Check sheet for the modelled part. Datum: model origin and axes. Units: mm. A direction names the side the tool comes from. Give positions to 0.01 mm unless a question says otherwise; leave off trailing zeros. Order: outer loops, then holes, each group sorted by start corner. A loop starts at its lowest first (then second) coordinate and runs counter-clockwise, first axis right, second up.
```python
from build123d import *

# Parameters (mm, degrees)
SKETCH1_R           = 69.85
BOSS_EXTRUDE1_DEPTH = 177.8
SKETCH2_R           = 25.4
CUT_EXTRUDE1_DEPTH  = 204.398340701
SKETCH3_R           = 63.5
CUT_EXTRUDE2_DEPTH  = 165.1


with BuildPart() as part:
    # Sketch1 → Boss-Extrude1 (new body)
    with BuildSketch(Plane.XY):
        Circle(SKETCH1_R)
    extrude(amount=BOSS_EXTRUDE1_DEPTH)

    # Sketch2 → Cut-Extrude1 (cut, through all)
    with BuildSketch(Plane.XY.offset(177.8)):
        Circle(SKETCH2_R)
    extrude(amount=-CUT_EXTRUDE1_DEPTH, mode=Mode.SUBTRACT)

    # Sketch3 → Cut-Extrude2 (cut)
    with BuildSketch(Plane.XY.offset(177.8)):
        Circle(SKETCH3_R)
    extrude(amount=-CUT_EXTRUDE2_DEPTH, mode=Mode.SUBTRACT)


solid = part.part
```
(1) Cross-section at A-A on x = 0. Enter the section's corners in (y, z).
Response values:
outline: (-69.85, 0) - (-25.4, 0) - (-25.4, 12.7) - (-63.5, 12.7) - (-63.5, 177.8) - (-69.85, 177.8) - close; (25.4, 0) - (69.85, 0) - (69.85, 177.8) - (63.5, 177.8) - (63.5, 12.7) - (25.4, 12.7) - close
(2) Release check for a two-part mould opening along X. For faces 1 (the face through (30, 1, 0)), 2 (the face through (-55.431, -42.503, 87.655)), 3 (the face through (27, 1, 12.7)) record: released by +X, released by -X, zero draft, split by the parting line, or undercut.
Response values:
face 1: zero draft
face 2: split by the parting line
face 3: undercut
(3) Set-up check for faces 4 (the face through (15, -62, 177.8)), 5 (the face through (-13.77, -61.99, 96.41)): record each of +Z, -Z, +X, -X, +Y, -Y from which the full face is reachable in a straight line by a thin tool's end or side.
Response values:
face 4: +Z, +X, -X, +Y, -Y
face 5: +Z
(4) Cross-section at D-D on y = -39.5. Enter the section's corners in (x, z).
Response values:
outline: (-57.61, 0) - (57.61, 0) - (57.61, 177.8) - (49.72, 177.8) - (49.72, 12.7) - (-49.72, 12.7) - (-49.72, 177.8) - (-57.61, 177.8) - close
(5) Gauge pin test, flat ends, axial feed: pin 1 Ø1 at (x, z) = (-27.5, 145) entering from +Y; pin 2 Ø6 at (x, z) = (47, 19) entering from -Y; pin 3 Ø4 at (x, z) = (-25, 147) entering from -Y. Record the tip position at first contact, or that the pin passes through.
Response values:
pin 1: stops at y = 64.42
pin 2: stops at y = -54.25
pin 3: stops at y = -65.95
(6) Material ranges on L1, parallel to X at y = -1.5, z = 105; L2, parallel to Y at x = 2.5, z = 80.5; L3, parallel to Y at x = 0, z = 80, recorded low to high.
Response values:
L1: x = -69.83 to -63.48, 63.48 to 69.83
L2: y = -69.81 to -63.45, 63.45 to 69.81
L3: y = -69.85 to -63.5, 63.5 to 69.85
(7) Cross-section at C-C on z = 128. Enter the section's corners in (x, y).
Response values:
outline: circle Ø139.7 at (0, 0); hole circle Ø127 at (0, 0)
